Work out the finished part from the listing and answer in its coordinate system (mm). A direction names the side the tool comes from. Coordinates: 2 decimals unless noted, no trailing zeros. Loops run counter-clockwise (first coordinate to the right, second up) from the corner with the lowest first, then second, coordinate; pieces in that order, holes last. Notation, with made-up numbers: (86, 30.25) - (123, 30.25) arc R19 ccw to (123, 66.25) - close; hole circle Ø8 at (11.25, -27.75). An arc over 180 degrees is marked (long way). Write each question's results on one line, items separated by ' | '. Start each with the question number.
Item 1: Each of these flat-tipped pins is pushed along its axis until it touches: pin 1 Ø10 at (x, y) = (205.5, -6) entering from -Z; pin 2 Ø1.1 at (y, z) = (-4, 5) entering from +X; pin 3 Ø1.1 at (x, z) = (201, 5) entering from +Y. Where does it stop, or does it pass through?
Item 2: Consider probe 1 along X at (y, z) = (-1, 9.75). Determine where the line is inside the solid, lowest interval first. Write a range as [from, to].
Item 3: A tool of negligible diameter and unlimited length cuts with its end or side. For faces 1 (the face through (205, -8, 4.5)), 2 (the face through (205, -16, 5.5)), 3 (the face through (3, -200, 5)), from which of +Z, -Z, +X, -X, +Y, -Y can it reach the whole face along a straight path? Write none if from no direction.
Item 4: Section A-A, the plane y = -49.5 is taken. Write down the section's boundary in (x, z).
Item 5: Section B-B, the plane z = 7.5 is taken. Write down the section's boundary in (x, y).
Autodesk Inventor part; units mm, degrees
ref_plane "YZ Plane" through (0, 0, 0) normal (1, 0, 0) x (0, 1, 0)
ref_plane "XZ Plane" through (0, 0, 0) normal (0, 1, 0) x (-1, 0, 0)
ref_plane "XY Plane" through (0, 0, 0) normal (0, 0, 1) x (1, 0, 0)
sketch "Skizze1" plane through (0, 0, 0) normal (0, 0, 1) x (1, 0, 0)
  line L0 (-200, 200) -> (200, 200)
  line L1 (200, 200) -> (200, -200)
  line L2 (200, -200) -> (-200, -200)
  line L3 (-200, -200) -> (-200, 200)
  line L4 (-280, 0) -> (280, 0)
  line L5 (0, -280) -> (0, 280)
  point P0 (0, 0)
  dimension "d0" = 400
  dimension "d1" = 400
extrude "Extrusion1" add sketch "Skizze1" along normal blind 10
sketch "Skizze2" plane through (200, -200, 0) normal (1, 0, 0) x (0, 0, -1)
  line L0 (0, 400) -> (0, 0)
  line L1 (0, 400) -> (-10, 400)
  line L2 (-10, 0) -> (-10, 400)
  line L3 (0, 0) -> (-10, 0)
  line L4 (-5.5, 182.5) -> (-4.5, 182.5)
  line L5 (-4.5, 182.5) -> (-4.5, 193.5)
  line L6 (-4.5, 193.5) -> (-5.5, 193.5)
  line L7 (-5.5, 193.5) -> (-5.5, 182.5)
  line L8 (-5.5, 182.5) -> (-4.5, 182.5)
  line L9 (-4.5, 182.5) -> (-4.5, 187)
  line L10 (-4.5, 187) -> (-5.5, 187)
  line L11 (-5.5, 187) -> (-5.5, 182.5)
  line L12 (-5.5, 189) -> (-4.5, 189)
  line L13 (-4.5, 189) -> (-4.5, 193.5)
  line L14 (-4.5, 193.5) -> (-5.5, 193.5)
  line L15 (-5.5, 193.5) -> (-5.5, 189)
  line L16 (-5.5, 182.5) -> (-4.5, 182.5)
  line L17 (-4.5, 182.5) -> (-4.5, 178)
  line L18 (-4.5, 178) -> (-5.5, 178)
  line L19 (-5.5, 178) -> (-5.5, 182.5)
  line L20 (-5.5, 193.5) -> (-4.5, 193.5)
  line L21 (-4.5, 193.5) -> (-4.5, 198)
  line L22 (-4.5, 198) -> (-5.5, 198)
  line L23 (-5.5, 198) -> (-5.5, 193.5)
  line L24 (-6.1285, 188) -> (-3.7092, 188)
  line L25 (-10, 0) -> (-10, 400)
  line L26 (0, 400) -> (0, 0)
  point P0 (0, 200)
  dimension "d4" = 20
  dimension "d5" = 1
  dimension "d6" = 11
  dimension "d7" = 2
  dimension "d8" = 4.5
  dimension "d10" = 178
extrude "Extrusion2" add sketch "Skizze2" along normal blind 4 contours L7 L10 L5 L4 | L4 L17 L18 L19 | L7 L6 L5 L12 | L23 L22 L21 L6
extrude "Extrusion4" add sketch "Skizze2" along normal blind 13 contours L7 L10 L5 L4 | L7 L6 L5 L12
pattern_linear "Rechteckige Anordnung1" count 2 spacing 27 along (0, 1, 0) of "Extrusion4", "Extrusion2"
properties part number "PV_Modul_CPY_3_CPY2" material "Glas"
Answer key:
1) pin 1: stops at z = 4.5 | pin 2: stops at x = 204 | pin 3: stops at y = 25
2) probe 1: x = [-200, 200]
3) face 1: -Z, +X, +Y, -Y | face 2: +Z, +X, +Y, -Y | face 3: +Z, -Z, +X, -X, -Y
4) outline: (-200, 0) - (200, 0) - (200, 10) - (-200, 10) - close
5) outline: (-200, -200) - (200, -200) - (200, 200) - (-200, 200) - close
